CAD build for the part. Positions are in the model's coordinates, mm. Face numbers are marked on the shaded views. Give positions to 0.01 mm unless a question says otherwise; leave off trailing zeros. Write each loop counter-clockwise with the first axis right and the second up, starting at its lowest first coordinate (ties: lowest second). Pieces come first, ordered by that corner, then holes. Notation, with made-up numbers: (-19, -28.75) -> (16, -28.75) arc R30 ccw to (16, -0.75) -> close; hole circle Ø8 at (24, -22). An arc over 180 degrees is marked (long way). Use one line per item in the form item = value. Start each with the question number.
Autodesk Inventor part; units mm, degrees
ref_plane "YZ Plane" through (0, 0, 0) normal (1, 0, 0) x (0, 1, 0)
ref_plane "XZ Plane" through (0, 0, 0) normal (0, 1, 0) x (-1, 0, 0)
ref_plane "XY Plane" through (0, 0, 0) normal (0, 0, 1) x (1, 0, 0)
sketch "Sketch2" plane through (0, 0, 0) normal (1, 0, 0) x (0, 1, 0)
  line L0 (75, 25) -> (-75, 25)
  line L1 (-75, 25) -> (-75, -25)
  line L2 (-75, -25) -> (75, -25)
  line L3 (75, -25) -> (75, 25)
  line L4 (75, 25) -> (-75, -25) construction
  line L5 (-75, 25) -> (75, -25) construction
  point P0 (0, 0)
  dimension "d4" = 150
  dimension "d5" = 50
extrude "Extrusion" add sketch "Sketch2" along normal blind 10
sketch "Sketch3" plane through (10, 0, 0) normal (1, 0, 0) x (0, 0, -1)
  circle A0 centre (-15, -45) radius 3.2
  circle A1 centre (15, -45) radius 3.2
  circle A2 centre (0, 60) radius 6.35
  point P0 (0, 0)
  dimension "d8" = 6.4
  dimension "d9" = 12.7
  dimension "d12" = 6.4
extrude "Extrusion2" cut sketch "Sketch3" against normal through all
properties part number "Stand"
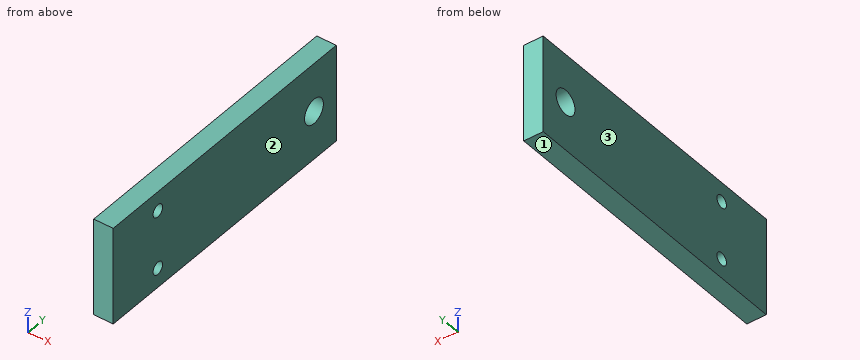
1) Cut at A-A (y = 60). Give the cut face in (x, z).
2) Cut at D-D (y = -45). Give the cut face in (x, z), and give its area (3 significant figures).
3) Pin check, flat tip, straight feed: pin 1 (8 mm diameter, centred on y = -33.5, z = -19.5, fed in from -X). Stop position of the tip, or through.
4) Wall check: line 1 along Y through (x, z) = (7, 15); line 2 along Y through (x, z) = (4.75, 0); line 3 along Z through (x, y) = (6.25, -47.5). Give the ranges that are in metal, low to high. Write a range as from..to.
5) Two-plate mould, pull along X, no slides. Class the marked faces 1, 2 and 3: released by +X, released by -X, zero draft, split by the parting line, or undercut.
6) Cut at B-B (x = 6). Give the cut face in (y, z), and give its area (3 significant figures).
7) Cut at C-C (z = 15). Give the cut face in (x, y).
Final values:
q1.outline = (0, -25) -> (10, -25) -> (10, -6.35) -> (0, -6.35) -> close; (0, 6.35) -> (10, 6.35) -> (10, 25) -> (0, 25) -> close
q2.outline = (0, -25) -> (10, -25) -> (10, -18.2) -> (0, -18.2) -> close; (0, -11.8) -> (10, -11.8) -> (10, 11.8) -> (0, 11.8) -> close; (0, 18.2) -> (10, 18.2) -> (10, 25) -> (0, 25) -> close
q2.area = 372 mm^2
q3.pin_1 = 0
q4.line_1 = -75..-48.2, -41.8..75
q4.line_2 = -75..53.65, 66.35..75
q4.line_3 = -25..-17, -13..13, 17..25
q5.face_1 = zero draft
q5.face_2 = released by +X
q5.face_3 = released by -X
q6.outline = (-75, -25) -> (75, -25) -> (75, 25) -> (-75, 25) -> close; hole circle Ø6.4 at (-45, -15); hole circle Ø6.4 at (-45, 15); hole circle Ø12.7 at (60, 0)
q6.area = 7,310 mm^2
q7.outline = (0, -75) -> (10, -75) -> (10, -48.2) -> (0, -48.2) -> close; (0, -41.8) -> (10, -41.8) -> (10, 75) -> (0, 75) -> close
